Part model, mm, in its own coordinate system. Face numbers are marked on the shaded views. A direction names the side the tool comes from. Coordinates: 2 decimals unless noted, no trailing zeros. Order: outer loops, then holes, each group sorted by start corner. A loop starts at its lowest first (then second) coordinate and runs counter-clockwise, first axis right, second up. Notation, with made-up numbers: (23.25, 69.25) - (40.25, 69.25) arc R16 ccw to (40.25, 77.25) - close; hole circle Ø11 at (58, -2). An arc over 180 degrees is marked (long way). Use a Markdown table: item, result. Add a question column.
1) Saw through at B-B on z = 8.25. List the corners of the cut face in (x, y), then the cut area to 3 significant figures.
2) Drop flat-ended pins along their axis: P1, Ø4.5, axis at x = 7.75, y = 8.5, coming from the -Z side; P2, Ø1.6, axis at y = 8, z = 9.5, coming from the -X side. Give the stop position or say it passes through.
3) Two-plate mould, pull along Y, no slides. Class the marked faces 4, 5 and 6: +Y half, -Y half, draft (parallel to the pull), parting line (faces both ways), or undercut.
4) Saw through at C-C on x = 7.75. Count the separate pieces of the cut face and the enclosed holes in it, then the cut area to 3 significant figures.
5) Saw through at A-A on y = 8.5. List the corners of the cut face in (x, z).
6) Wall check: L1, parallel to Y at x = 7.75, z = 7; L2, parallel to Y at x = 7.75, z = 1.2; L3, parallel to Y at x = 1.5, z = 12.25. Give the ranges that are in metal, low to high. Write a range as [from, to].
7) Tool access for the marked faces 1, 2 and 3: list every direction of +Z, -Z, +X, -X, +Y, -Y with a clear straight run to the whole face (end or side of a thin tool).
```python
from build123d import *

# Parameters (mm, degrees)
F0_R     = 1.7
F1_DEPTH = 14
F2_R     = 2.88
F2_R_2   = 1.7
F3_DEPTH = 3
F4_R     = 0.55
F5_DEPTH = 7
F6_R     = 0.45


with BuildPart() as f1:
    # F0 (on Top) → F1 (new body)
    with BuildSketch(Plane.XY):
        Polygon((0, 6.89), (0, 0), (12, 0), (12, 3), (5, 3), (5, 3.76), (12, 3.76), (12, 11.8), (0, 11.8), (0, 10.1), (2.1, 10.1), (2.1, 6.89), align=None)
        with Locations((7.75, 8.5)):
            Circle(F0_R, mode=Mode.SUBTRACT)
    extrude(amount=F1_DEPTH)

    # F2 (on face) → F3 (cut)
    with BuildSketch(Plane(origin=(0, 0, 0), x_dir=(1, 0, 0), z_dir=(0, 0, -1))):
        with Locations((7.75, -8.5)):
            Circle(F2_R)
        with Locations((7.75, -8.5)):
            Circle(F2_R_2, mode=Mode.SUBTRACT)
    extrude(amount=-F3_DEPTH, mode=Mode.SUBTRACT)

    # F4 (on face) → F5 (cut, through all)
    with BuildSketch(Plane.YZ.offset(12)):
        with Locations((3.98, 12.88)):
            Circle(F4_R)
        with Locations((3.98, 10.93)):
            Circle(F4_R)
        with Locations((3.98, 8.98)):
            Circle(F4_R)
        with Locations((3.98, 7.03)):
            Circle(F4_R)
        with Locations((3.98, 5.08)):
            Circle(F4_R)
        with Locations((3.98, 3.13)):
            Circle(F4_R)
        with Locations((3.98, 1.18)):
            Circle(F4_R)
    extrude(amount=-F5_DEPTH, mode=Mode.SUBTRACT)

    # F6
    f6_edges = [f1.edges().sort_by_distance(p)[0] for p in [
        (8.5, 3.76, 12.375917),
        (8.5, 3.76, 13.384083),
        (8.5, 3.76, 11.434083),
        (8.5, 3.76, 10.425917),
        (8.5, 3.76, 9.484083),
        (8.5, 3.76, 8.475917),
        (8.5, 3.76, 7.534083),
        (8.5, 3.76, 6.525917),
        (8.5, 3.76, 5.584083),
        (8.5, 3.76, 4.575917),
        (8.5, 3.76, 3.634083),
        (8.5, 3.76, 2.625917),
        (8.5, 3.76, 1.684083),
        (8.5, 3.76, 0.675917),
    ]]
    fillet(f6_edges, radius=F6_R)


solid = f1.part
```
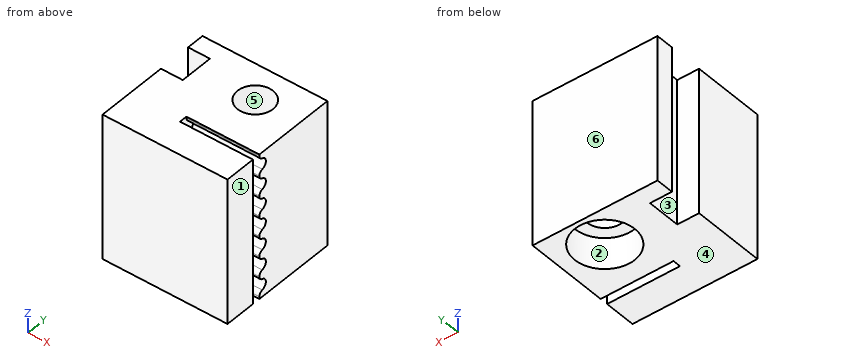
Results are:
| question | item | result |
|---|---|---|
| 1 | outline | (0, 0) - (12, 0) - (12, 3) - (5, 3) - (5, 3.83) - (12, 3.83) - (12, 11.8) - (0, 11.8) - (0, 10.1) - (2.1, 10.1) - (2.1, 6.89) - (0, 6.89) - close; hole circle Ø3.4 at (7.75, 8.5) |
| 1 | area | 120 mm2 |
| 2 | P1 | z = 3 |
| 2 | P2 | x = 2.1 |
| 3 | face 4 | draft |
| 3 | face 5 | undercut |
| 3 | face 6 | +Y half |
| 4 | separate pieces | 3 |
| 4 | enclosed holes | 0 |
| 4 | area | 94.4 mm2 |
| 5 | outline | (2.1, 0) - (4.87, 0) - (4.87, 3) - (6.05, 3) - (6.05, 14) - (2.1, 14) - close; (9.45, 3) - (10.63, 3) - (10.63, 0) - (12, 0) - (12, 14) - (9.45, 14) - close |
| 6 | L1 | [0, 3], [4.53, 6.8], [10.2, 11.8] |
| 6 | L2 | [0, 3], [4.53, 5.62], [11.38, 11.8] |
| 6 | L3 | [0, 6.89], [10.1, 11.8] |
| 7 | face 1 | +Z, -Z, +X, +Y, -Y |
| 7 | face 2 | -Z |
| 7 | face 3 | +Z, -Z, -X |
